Here's the drawing with two shaded views (mm, measured from the low corner). I have some questions. A direction names the side the tool comes from. Give positions to 0.01 mm unless a question says otherwise; leave off trailing zeros. Loops run counter-clockwise (first coordinate to the right, second up) from the corner with the lowest first, then second, coordinate; pieces in that order, holes last. Notation, with made-up numbers: (47, 28) - (79, 28) arc R21 ccw to (79, 47) - close; hole circle Ø8 at (-8, 47). An arc over 180 degrees is marked (long way). Answer as a JSON object with one key per item and string values. Group by question number.
Item 1: Please list where these lines run through material, in increasing order: L1, parallel to X at y = 13, z = 7.5; L2, parallel to X at y = 5, z = 3.25; L3, parallel to Z at x = 26.5, y = 3.25.
Item 2: Will these pins go through, and if not, where does the flat tip stop? pin 1 (1.5 mm diameter, centred on y = 15.5, z = 2.5, fed in from -X); pin 2 (1 mm diameter, centred on x = 29.5, z = 4.5, fed in from -Y); pin 3 (10.5 mm diameter, centred on x = 15.5, y = 6, fed in from +Z); pin 4 (10 mm diameter, centred on x = 12, y = 12.5, fed in from -Z).
Item 3: Which directions (+Z, -Z, +X, -X, +Y, -Y) give clear straight access to the entire face, cutting with the end or side of a thin tool? Please do the marked faces 1, 2 and 3.
Item 4: Suppose I cut it at C-C on z = 7. Write out the boundary of the cut face in (x, y).
Item 5: Suppose I cut it at B-B on y = 15.5. Write out the boundary of the cut face in (x, z).
Item 6: Thinking about a two-plate mould opening in X: for the marked faces 4, 5, 6 and 7, which applies, pulls with the +X half, pulls with the -X half, needs draft (parallel to the pull), parting line crosses it, or undercut?
Item 7: Suppose I cut it at A-A on z = 4.5. Write out the boundary of the cut face in (x, y).
Item 8: Suppose I cut it at D-D on x = 4. Write out the boundary of the cut face in (y, z), and give its area (3 significant figures).
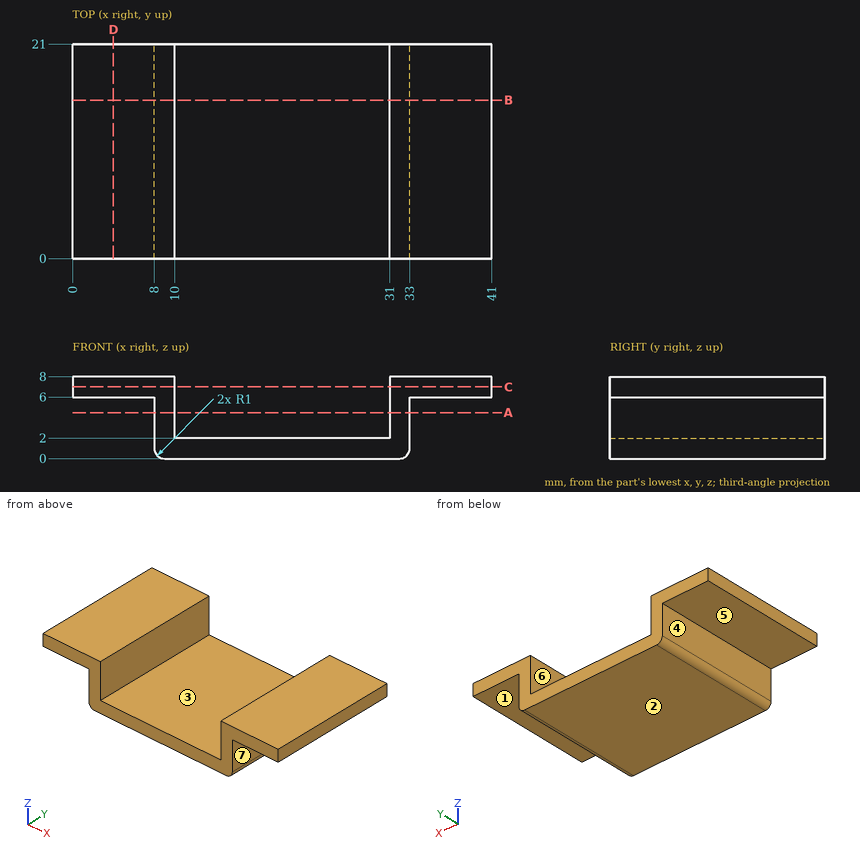
Worked out:
{
 "1": {"L1": "x = 0 to 10, 31 to 41", "L2": "x = 8 to 10, 31 to 33", "L3": "z = 0 to 2"},
 "2": {"pin 1": "stops at x = 8", "pin 2": "passes through", "pin 3": "stops at z = 2", "pin 4": "stops at z = 0"},
 "3": {"face 1": "-Z, +X, +Y, -Y", "face 2": "-Z, +X, -X, +Y, -Y", "face 3": "+Z, +Y, -Y"},
 "4": {"outline": "(0, 0) - (10, 0) - (10, 21) - (0, 21) - close; (31, 0) - (41, 0) - (41, 21) - (31, 21) - close"},
 "5": {"outline": "(0, 6) - (8, 6) - (8, 1) arc R1 ccw to (9, 0) - (32, 0) arc R1 ccw to (33, 1) - (33, 6) - (41, 6) - (41, 8) - (31, 8) - (31, 2) - (10, 2) - (10, 8) - (0, 8) - close"},
 "6": {"face 4": "pulls with the -X half", "face 5": "needs draft", "face 6": "undercut", "face 7": "pulls with the +X half"},
 "7": {"outline": "(8, 0) - (10, 0) - (10, 21) - (8, 21) - close; (31, 0) - (33, 0) - (33, 21) - (31, 21) - close"},
 "8": {"outline": "(0, 6) - (21, 6) - (21, 8) - (0, 8) - close", "area": "42.0 mm2"}
}
